For this review, take the finished solid that the model builds, in its own axes (mm). Coordinates: 2 decimals unless noted, no trailing zeros. Write each loop counter-clockwise with the first axis right and the second up, starting at its lowest first coordinate (ties: lowest second). Pieces come first, ordered by that corner, then holes.
1) We need section C-C on x = 146.5. Write out the cut boundary in (y, z), then the cut area to 3 significant figures.
2) We need section B-B on x = -157. Write out the cut boundary in (y, z).
3) To check wall thickness, follow line 1 along Y through (x, z) = (0, 1.2); line 2 along X through (y, z) = (78.5, 1.5); line 3 along Y through (x, z) = (123, 0.8). State the ranges of each line that lie inside material, in increasing order.
4) We need section A-A on z = 0.9. Give the number of separate pieces and of enclosed holes in the cut face, then the cut area to 3 significant figures.
5) Insertion check: P1, Ø1, axis at x = -137, z = 0.5, coming from the -Y side; P2, Ø0.6, axis at y = 66, z = 1, coming from the -X side; P3, Ø1, axis at y = -7, z = 0.5, coming from the -X side. Each pin has a flat end and moves straight along its axis. Give the tip position at first contact, or say it passes through.
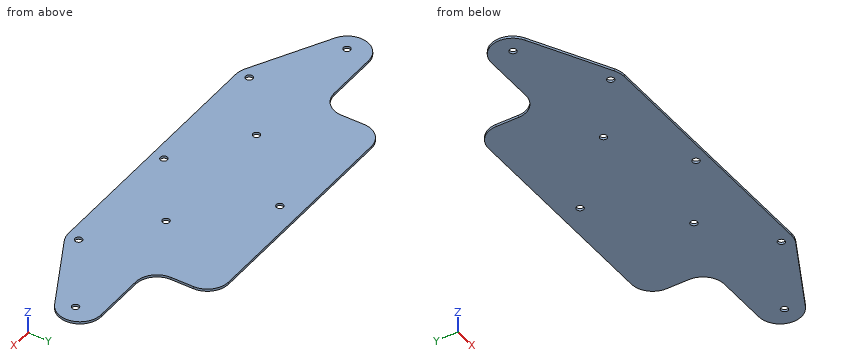
from build123d import *

# Parameters (mm, degrees)
ESQUISSE1_R        = 3
BOSS_EXTRU_1_DEPTH = 2
CONG_1_R           = 18
CONG_2_R           = 20


with BuildPart() as part:
    # Esquisse1 → Boss.-Extru.1 (new body)
    with BuildSketch(Plane.XY):
        Polygon((-244.958991582, 40), (-110, 40), (-110, 95), (110, 95), (110, 40), (244.958991582, 40), (112.479495791, -30), (-112.479495791, -30), align=None)
        with Locations((-175, 20)):
            Circle(ESQUISSE1_R, mode=Mode.SUBTRACT)
        with Locations((-110, -20)):
            Circle(ESQUISSE1_R, mode=Mode.SUBTRACT)
        with Locations((110, -20)):
            Circle(ESQUISSE1_R, mode=Mode.SUBTRACT)
        with Locations((175, 20)):
            Circle(ESQUISSE1_R, mode=Mode.SUBTRACT)
        with Locations((0, -20)):
            Circle(ESQUISSE1_R, mode=Mode.SUBTRACT)
        with Locations((-58.333333333, 20)):
            Circle(ESQUISSE1_R, mode=Mode.SUBTRACT)
        with Locations((58.333333333, 20)):
            Circle(ESQUISSE1_R, mode=Mode.SUBTRACT)
        with Locations((0, 78.03)):
            Circle(ESQUISSE1_R, mode=Mode.SUBTRACT)
    extrude(amount=BOSS_EXTRU_1_DEPTH)

    # Congé1
    cong_1_edges = [part.edges().sort_by_distance(p)[0] for p in [
        (-244.958991582, 40, 1),
        (-110, 40, 1),
        (-110, 95, 1),
        (110, 95, 1),
        (110, 40, 1),
        (244.958991582, 40, 1),
    ]]
    fillet(cong_1_edges, radius=CONG_1_R)

    # Congé2
    cong_2_edges = [part.edges().sort_by_distance(p)[0] for p in [
        (112.479495791, -30, 1),
        (-112.479495791, -30, 1),
    ]]
    fillet(cong_2_edges, radius=CONG_2_R)


solid = part.part
Result:
1. outline: (-12.02, 0) - (40, 0) - (40, 2) - (-12.02, 2) - close
1. area: 104 mm2
2. outline: (-6.48, 0) - (40, 0) - (40, 2) - (-6.48, 2) - close
3. line 1: y = -30 to -23, -17 to 75.03, 81.03 to 95
3. line 2: x = -109.94 to -2.96, 2.96 to 109.94
3. line 3: y = -24.44 to 40.71
4. separate pieces: 1
4. enclosed holes: 8
4. area: 35,100 mm2
5. P1: stops at y = -17.31
5. P2: stops at x = -110
5. P3: stops at x = -156.95
